```python
from build123d import *

# Parameters (mm, degrees)
CUT_EXTRUDE_1_DEPTH = 1.5
FILLET_1_R          = 0.3
CHAMFER_1_SIZE      = 0.5


with BuildPart() as part:
    # Эскиз1 → Повернуть1 (revolve)
    with BuildSketch(Plane.XY, mode=Mode.PRIVATE) as revolve_1_sk:
        with BuildLine():
            Line((0, 0), (0, 2.875))
            ThreePointArc((0, 2.875), (0.908484425, 3.521678457), (2, 3.75))
            Line((2, 3.75), (2.5, 3.75))
            Line((2.5, 3.75), (2.5, 2))
            Line((2.5, 2), (10.5, 2))
            Line((10.5, 2), (10.5, 0))
            Line((10.5, 0), (0, 0))
        make_face()
    revolve(revolve_1_sk.sketch.rotate(Axis((10.5, 0, 0), (-1, 0, 0)), 90), axis=Axis((10.5, 0, 0), (-1, 0, 0)))  # turned: the seam where the file's is

    # Эскиз2 → Вырез-Вытянуть1 (cut)
    with BuildSketch(Plane.ZY):
        Polygon((0.721687836, 1.25), (-0.721687836, 1.25), (-1.443375673, 0), (-0.721687836, -1.25), (0.721687836, -1.25), (1.443375673, 0), align=None)
    extrude(amount=-CUT_EXTRUDE_1_DEPTH, mode=Mode.SUBTRACT)

    # Скругление1
    fillet_1_edges = [part.edges().sort_by_distance(p)[0] for p in [
        (2.5, 0, 2),
        (2.5, 0, 3.75),
    ]]
    fillet(fillet_1_edges, radius=FILLET_1_R)

    # Фаска1
    chamfer_1_edges = [part.edges().sort_by_distance(p)[0] for p in [
        (10.5, 0, 2),
    ]]
    chamfer(chamfer_1_edges, length=CHAMFER_1_SIZE)


solid = part.part
```
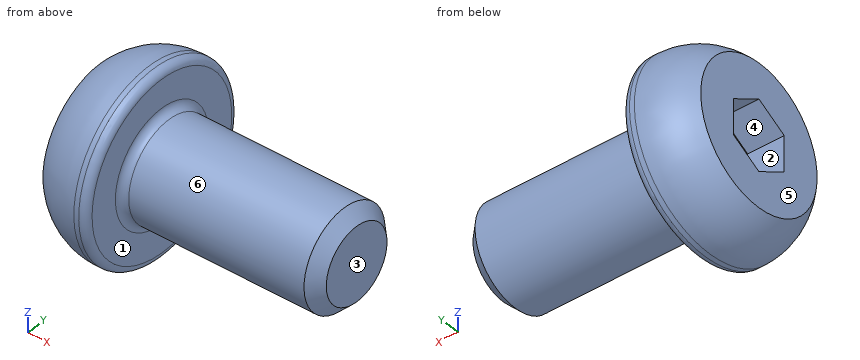
The listing builds one solid part. Answer for the finished solid, in the listing's coordinates (mm). Face numbers are marked on the shaded views. A direction names the side the tool comes from. Round coordinates to 2 decimals unless told otherwise and drop trailing zeros. Loops run counter-clockwise (first coordinate to the right, second up) from the corner with the lowest first, then second, coordinate; pieces in that order, holes last. Notation, with made-up numbers: (46.25, -17.75) - (64.25, -17.75) arc R14 ccw to (64.25, -0.75) - close; hole circle Ø5 at (78.25, 11). An arc over 180 degrees is marked (long way). Return JSON: item names as keys, results as strings. Group by question number.
1. The part is cut by section A-A on x = 8.25. Determine the outline of the cut face in (y, z).
2. The mould has two halves that part along Z. Classify the marked faces 4, 5 and 6: pulls with the +Z half, pulls with the -Z half, needs draft (parallel to the pull), parting line crosses it, or undercut.
3. Consider probe 1 along X at (y, z) = (0.75, 0.5); probe 2 along X at (y, z) = (-2.5, -0.75); probe 3 along Z at (x, y) = (7.5, -0.5). Determine where each line is inside the solid, lowest interval first.
4. Which of the six approach directions +Z, -Z, +X, -X, +Y, -Y give full straight-line access (tool end or side, diameter ignored) to the marked faces 1, 2 and 3?
5. Each of these flat-tipped pins is pushed along its axis until it touches: P1, Ø3, axis at y = -0.5, z = 0, coming from the -X side; P2, Ø4, axis at x = 3, z = 2.5, coming from the +Y side; P3, Ø1.2, axis at x = 0.5, z = 0, coming from the -Y side; P4, Ø3, axis at x = 4.5, z = -2.5, coming from the +Y side. Where does it stop, or does it pass through?
Resolved:
{
 "1": {"outline": "circle Ø4 at (0, 0)"},
 "2": {"face 4": "undercut", "face 5": "needs draft", "face 6": "parting line crosses it"},
 "3": {"probe 1": "x = 1.5 to 10.5", "probe 2": "x = 0 to 2.5", "probe 3": "z = -1.94 to 1.94"},
 "4": {"face 1": "+X", "face 2": "-X", "face 3": "+Z, -Z, +X, +Y, -Y"},
 "5": {"P1": "stops at x = 0", "P2": "stops at y = 3.69", "P3": "stops at y = -3.6", "P4": "stops at y = 1.73"}
}
